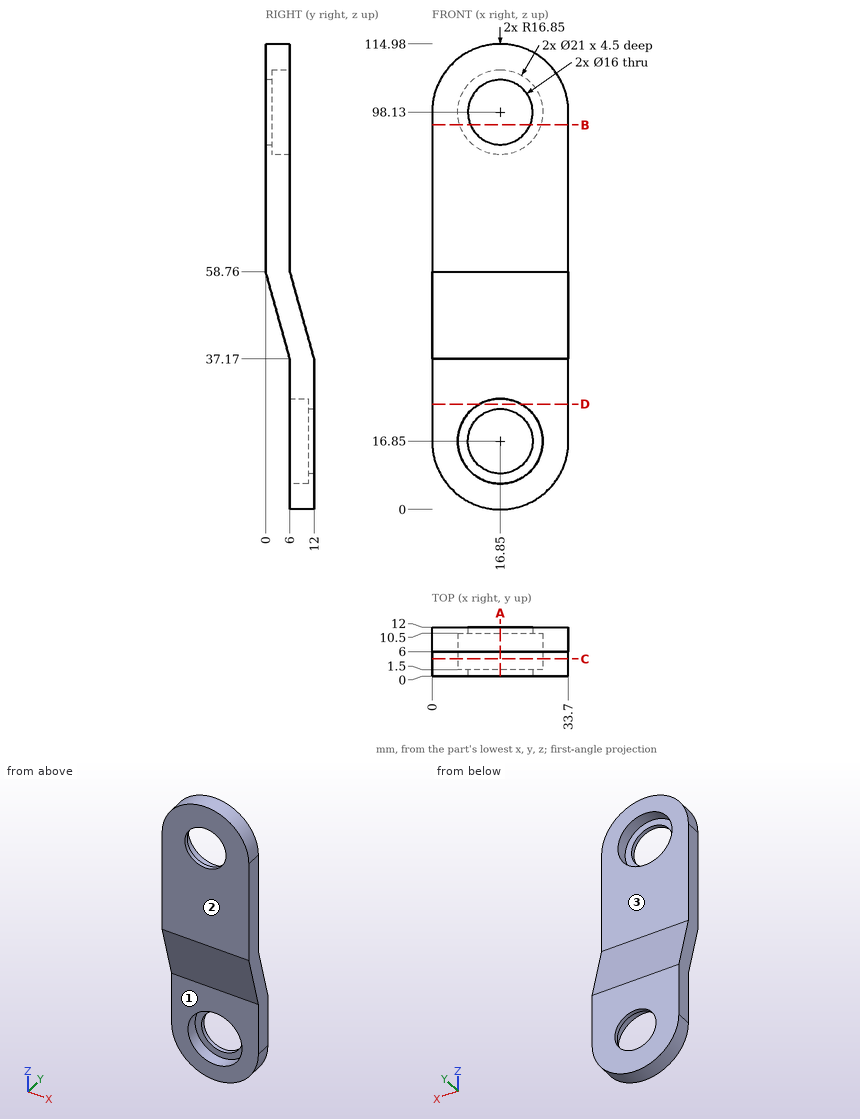
Source: three-view drawing plus pictorial views. Frame: mm from the lowest corner of the part. A direction names the side the tool comes from. Coordinates: 2 decimals unless noted, no trailing zeros. Write each loop counter-clockwise with the first axis right and the second up, starting at its lowest first coordinate (ties: lowest second). Pieces come first, ordered by that corner, then holes. Notation, with made-up numbers: (-14.5, 47.5) -> (-10.5, 47.5) arc R24 cw to (-10.5, 73.5) -> close; hole circle Ø9 at (32, 43). An arc over 180 degrees is marked (long way). Answer as a JSON object with one key per item and string values.
1. Section D-D on z = 26. Return the cut outline in (x, y).
Result set:
{"outline": "(0, 6) -> (11.7, 6) -> (11.7, 10.5) -> (22, 10.5) -> (22, 6) -> (33.7, 6) -> (33.7, 12) -> (0, 12) -> close"}
2. Access query for the marked faces 1, 2 and 3. Directions: +Z, -Z, +X, -X, +Y, -Y. A direction counts if a zero-diameter tool reaches every point of the face in a straight line with its end or side. Return the directions, or none.
Result set:
{"face 1": "-Z, +X, -X, -Y", "face 2": "+Z, -Z, +X, -X, -Y", "face 3": "+Z, +X, -X, +Y"}
3. Section A-A on x = 16.85. Return the cut outline in (y, z), then the cut area to 3 significant figures.
Result set:
{"outline": "(0, 58.76) -> (6, 37.17) -> (6, 27.35) -> (10.5, 27.35) -> (10.5, 24.85) -> (12, 24.85) -> (12, 37.17) -> (6, 58.76) -> (6, 87.63) -> (1.5, 87.63) -> (1.5, 90.13) -> (0, 90.13) -> close; (0, 106.13) -> (1.5, 106.13) -> (1.5, 108.63) -> (6, 108.63) -> (6, 114.98) -> (0, 114.98) -> close; (6, 0) -> (12, 0) -> (12, 8.85) -> (10.5, 8.85) -> (10.5, 6.35) -> (6, 6.35) -> close", "area": "453 mm2"}
4. Section B-B on z = 95. Return the cut outline in (x, y).
Result set:
{"outline": "(0, 0) -> (9.49, 0) -> (9.49, 1.5) -> (6.83, 1.5) -> (6.83, 6) -> (0, 6) -> close; (24.21, 0) -> (33.7, 0) -> (33.7, 6) -> (26.87, 6) -> (26.87, 1.5) -> (24.21, 1.5) -> close"}
5. Material intervals for line 1 (X direction, y = 8.5, z = 16.85); line 2 (X direction, y = 0.5, z = 98.13); line 3 (Y direction, x = 5, z = 12.5), sorted ascending. Write a range as from..to.
Result set:
{"line 1": "x = 0..6.35, 27.35..33.7", "line 2": "x = 0..8.85, 24.85..33.7", "line 3": "y = 6..12"}
6. First-contact query: P1, Ø17, axis at x = 11.5, z = 83.5, coming from the +Y side; P2, Ø1, axis at x = 29, z = 45, coming from the -Y side; P3, Ø5, axis at x = 8, y = 7.5, coming from the -Z side. Flat tips, straight axial feed; report the tip coordinate or a pass-through.
Result set:
{"P1": "stops at y = 6", "P2": "stops at y = 3.69", "P3": "stops at z = 1.24"}
7. Section C-C on y = 4.25. Return the cut outline in (x, z), then the cut area to 3 significant figures.
Result set:
{"outline": "(0, 43.47) -> (33.7, 43.47) -> (33.7, 98.13) arc R16.85 ccw to (0, 98.13) -> close; hole circle Ø21 at (16.85, 98.13)", "area": "1,940 mm2"}
